Here's the drawing with two shaded views (mm, measured from the low corner). I have some questions. A direction names the side the tool comes from. Coordinates: 2 decimals unless noted, no trailing zeros. Order: outer loops, then holes, each group sorted by start corner. A loop starts at its lowest first (then second) coordinate and runs counter-clockwise, first axis right, second up. Notation, with made-up numbers: (-24.75, 64.5) -> (0.25, 64.5) arc R12 cw to (0.25, 72.5) -> close; hole circle Ø8 at (-1.75, -39). An arc over 180 degrees is marked (long way). Answer as a JSON object with one key per item and string values. Group by question number.
(1) Which directions (+Z, -Z, +X, -X, +Y, -Y) give clear straight access to the entire face, cutting with the end or side of a thin tool? Please do the marked faces 5, 6 and 7.
(2) I want a section at C-C, the plane z = 5.5. List the corners of the cut face in (x, y) for me.
(3) I want a section at B-B, the plane x = 18. List the corners of the cut face in (y, z) for me, plus the area to 4 significant figures.
(4) If we mould it in two halves opening along Z, with no side actions, what happens to the marked faces 1, 2, 3 and 4? For each: pulls with the +Z half, pulls with the -Z half, needs draft (parallel to the pull), parting line crosses it, or undercut.
(5) For pin 1 (3 mm diameter, centred on y = 12, z = 16, fed in from -X); pin 2 (1 mm diameter, centred on x = 22, z = 8, fed in from -Y); pin 3 (4 mm diameter, centred on y = 18.5, z = 3, fed in from -X), each with a flat end and sliding along its axis, tell me the tip position at first contact or that it passes through.
(6) I need wall thicknesses on line 1 (X direction, y = 18, z = 4.75); line 2 (Y direction, x = 18, z = 7.5). Which ranges of each line are inside material? Lowest first, please.
(7) I want a section at D-D, the plane y = 27.5. List the corners of the cut face in (x, z) for me, plus the area to 3 significant figures.
(8) I want a section at A-A, the plane y = 2. List the corners of the cut face in (x, z) for me, plus the area to 3 significant figures.
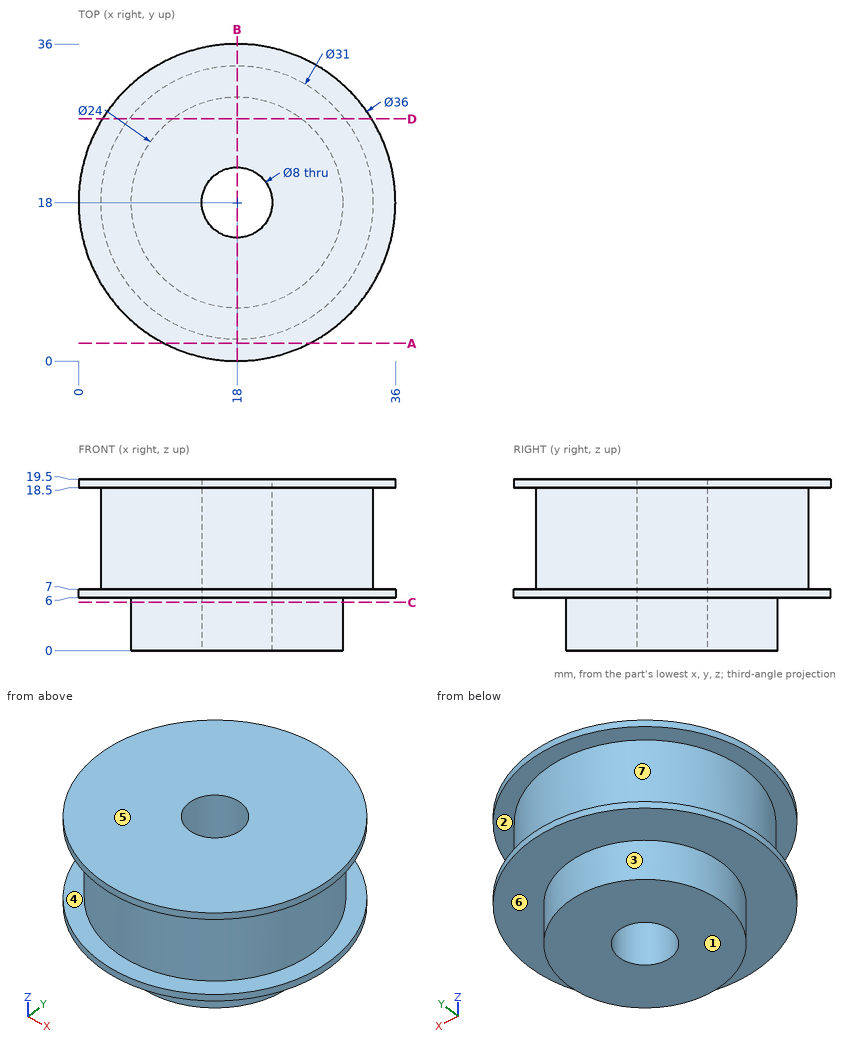
Computed values:
{
 "1": {"face 5": "+Z, +X, -X, +Y, -Y", "face 6": "-Z", "face 7": "none"},
 "2": {"outline": "circle Ø24 at (18, 18); hole circle Ø8 at (18, 18)"},
 "3": {"outline": "(0, 6) -> (6, 6) -> (6, 0) -> (14, 0) -> (14, 19.5) -> (0, 19.5) -> (0, 18.5) -> (2.5, 18.5) -> (2.5, 7) -> (0, 7) -> close; (22, 0) -> (30, 0) -> (30, 6) -> (36, 6) -> (36, 7) -> (33.5, 7) -> (33.5, 18.5) -> (36, 18.5) -> (36, 19.5) -> (22, 19.5) -> close", "area": "416.5 mm2"},
 "4": {"face 1": "pulls with the -Z half", "face 2": "undercut", "face 3": "needs draft", "face 4": "undercut"},
 "5": {"pin 1": "stops at x = 3.17", "pin 2": "stops at y = 2.9", "pin 3": "stops at x = 6"},
 "6": {"line 1": "x = 6 to 14, 22 to 30", "line 2": "y = 2.5 to 14, 22 to 33.5"},
 "7": {"outline": "(2.71, 6) -> (10.67, 6) -> (10.67, 0) -> (25.33, 0) -> (25.33, 6) -> (33.29, 6) -> (33.29, 7) -> (30.25, 7) -> (30.25, 18.5) -> (33.29, 18.5) -> (33.29, 19.5) -> (2.71, 19.5) -> (2.71, 18.5) -> (5.75, 18.5) -> (5.75, 7) -> (2.71, 7) -> close", "area": "431 mm2"},
 "8": {"outline": "(9.75, 6) -> (26.25, 6) -> (26.25, 7) -> (9.75, 7) -> close; (9.75, 18.5) -> (26.25, 18.5) -> (26.25, 19.5) -> (9.75, 19.5) -> close", "area": "33.0 mm2"}
}
